Can you work these out from the model? Positions are in its coordinate system, mm. Face numbers are marked on the shaded views. A direction names the side the tool comes from. Give positions to 0.01 mm unless a question says otherwise; leave off trailing zeros. Order: outer loops, then holes, each group sorted by start corner. A loop starts at its lowest first (then second) coordinate and runs counter-clockwise, first axis right, second up. Notation, with made-up numbers: M 55.25,25 L 86.25,25 A20 ccw 86.25,44 Z; hole C 18,-13.5 d9. An arc over 180 degrees is marked long. Use one line per item in the form item = value. Start each with the question number.
1. I want a section at B-B, the plane y = 1.5. List the corners of the cut face in (x, z) for me.
2. I need wall thicknesses on L1, parallel to X at y = -1.5, z = 5; L2, parallel to Z at x = 9.5, y = -1.75; L3, parallel to X at y = -1.75, z = 5. Which ranges of each line are inside material? Lowest first, please.
3. I want a section at A-A, the plane z = 5. List the corners of the cut face in (x, y) for me, and give its area (3 significant figures).
4. I want a section at C-C, the plane x = 0. List the corners of the cut face in (y, z) for me, and give its area (3 significant figures).
5. I want a section at D-D, the plane y = -4.5. List the corners of the cut face in (x, z) for me, and give its area (3 significant figures).
6. We'd pull the mould along Y, two halves only. Please class the marked faces 1, 2, 3 and 4: +Y half, -Y half, draft (parallel to the pull), parting line (faces both ways), or undercut.
7. Will these pins go through, and if not, where does the flat tip stop? P1, Ø4, axis at y = 4, z = 14, coming from the -X side; P2, Ø4, axis at x = 9, y = -2, coming from the +Z side; P3, Ø4, axis at x = 8, z = 1.5, coming from the -Y side.
8. For the marked faces 5, 6 and 7, which set-ups out of +Z, -Z, +X, -X, +Y, -Y let a thin tool reach every point of the face, with its end or its side?
```python
from build123d import *

# Parameters (mm, degrees)
SKETCH1_R                       = 4
MAIN_DEPTH                      = 10
SKETCH3_W                       = 20
SKETCH3_H                       = 2.9
MAKERBEAMRECTANGULARGUIDE_DEPTH = 1
SKETCH4_R                       = 1.5
MAKERBEAMFIXHOLE_DEPTH          = 9
FILLET1_R                       = 2
SKETCH5_R                       = 4
BOSS_EXTRUDE1_DEPTH             = 10


with BuildPart() as part:
    # Sketch1 → Main (new body)
    with BuildSketch(Plane.XY):
        with BuildLine():
            Line((-5.5, 0), (-5.5, -5))
            Line((-5.5, -5), (14.5, -5))
            Line((14.5, -5), (14.5, 2))
            Line((14.5, 2), (5.123475383, 2))
            ThreePointArc((5.123475383, 2), (-1.017567048, 5.405049242), (-5.5, 0))
        make_face()
        Circle(SKETCH1_R, mode=Mode.SUBTRACT)
    extrude(amount=MAIN_DEPTH)

    # Sketch3 → MakerBeamRectangularGuide (add)
    with BuildSketch(Plane(origin=(0, -5, 0), x_dir=(-1, 0, 0), z_dir=(0, -1, 0))):
        with Locations((-4.5, -5)):
            Rectangle(SKETCH3_W, SKETCH3_H)
    extrude(amount=MAKERBEAMRECTANGULARGUIDE_DEPTH)

    # Sketch4 → MakerBeamFixHole (cut, through all)
    with BuildSketch(Plane(origin=(0, 2, 0), x_dir=(1, 0, 0), z_dir=(0, 1, 0))):
        with Locations((9.5, -5)):
            Circle(SKETCH4_R)
    extrude(amount=-MAKERBEAMFIXHOLE_DEPTH, mode=Mode.SUBTRACT)

    # Fillet1
    fillet1_edges = [part.edges().sort_by_distance(p)[0] for p in [
        (5.123475383, 2, 5),
    ]]
    fillet(fillet1_edges, radius=FILLET1_R)

    # Sketch5 → Boss-Extrude1 (add)
    with BuildSketch(Plane.XY.offset(10)):
        with BuildLine():
            Line((-5.5, -5), (5.5, -5))
            Line((5.5, -5), (5.5, 0))
            ThreePointArc((5.5, 0), (0, 5.5), (-5.5, 0))
            Line((-5.5, 0), (-5.5, -5))
        make_face()
        Circle(SKETCH5_R, mode=Mode.SUBTRACT)
    extrude(amount=BOSS_EXTRUDE1_DEPTH)


solid = part.part
```
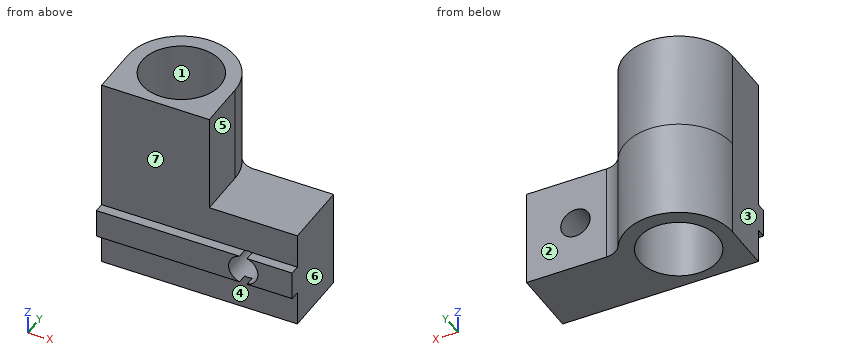
Check result:
q1.outline = M -5.29,0 L -3.71,0 L -3.71,20 L -5.29,20 Z; M 3.71,0 L 14.5,0 L 14.5,10 L 5.29,10 L 5.29,20 L 3.71,20 Z; hole C 9.5,5 d3
q2.L1 = -5.5 to -3.71, 3.71 to 8, 11 to 14.5
q2.L2 = 0 to 3.5, 6.5 to 10
q2.L3 = -5.5 to -3.6, 3.6 to 8, 11 to 14.5
q3.outline = M -5.5,-6 L 8,-6 L 8,2 L 6.34,2 A2 cw 4.65,2.93 A5.5 ccw -5.5,0 Z; M 11,-6 L 14.5,-6 L 14.5,2 L 11,2 Z; hole C 0,0 d8
q3.area = 112 mm2
q4.outline = M -6,3.55 L -5,3.55 L -5,0 L -4,0 L -4,20 L -5,20 L -5,6.45 L -6,6.45 Z; M 4,0 L 5.5,0 L 5.5,20 L 4,20 Z
q4.area = 52.9 mm2
q5.outline = M -5.5,0 L 14.5,0 L 14.5,10 L 5.5,10 L 5.5,20 L -5.5,20 Z; hole C 9.5,5 d3
q5.area = 303 mm2
q6.face_1 = undercut
q6.face_2 = +Y half
q6.face_3 = draft
q6.face_4 = -Y half
q7.P1 = -5.12
q7.P2 = 10
q7.P3 = -5
q8.face_5 = +Z, +X, +Y, -Y
q8.face_6 = +Z, -Z, +X, +Y, -Y
q8.face_7 = +Z, +X, -X, -Y
